from build123d import *
from build123d.topology import SkipClean

# Parameters (mm, degrees)
SKETCH1_R           = 17.5
BOSS_EXTRUDE1_DEPTH = 39
FILLET1_R           = 4.5
SKETCH2_R           = 5
BOSS_EXTRUDE2_DEPTH = 90
SKETCH6_W           = 6
SKETCH6_H           = 26
SKETCH6_W_2         = 14
SKETCH6_W_3         = 18.119457468
SKETCH6_H_2         = 239
SKETCH6_W_4         = 26
SKETCH6_H_3         = 15
SKETCH7_W           = 44.5
SKETCH7_H           = 15
SKETCH8_R           = 28.3
BOSS_EXTRUDE5_DEPTH = 6.5
SKETCH9_R           = 80
BOSS_EXTRUDE6_DEPTH = 1.8
BOSS_EXTRUDE7_START = 13.3
SKETCH10_R          = 8.5
SKETCH10_R_2        = 7.120417841
SKETCH10_R_3        = 5
BOSS_EXTRUDE7_DEPTH = 8
BOSS_EXTRUDE8_START = 21.3
SKETCH10_3_R        = 8.5
SKETCH10_3_R_2      = 7.120417841
SKETCH10_3_R_3      = 5
BOSS_EXTRUDE8_DEPTH = 8
SKETCH14_R          = 28.5
SKETCH14_R_2        = 19.5
BOSS_EXTRUDE9_DEPTH = 26.880542532


with BuildPart() as part:
    # Sketch1 → Boss-Extrude1 (new, symmetric)
    with BuildSketch(Plane(origin=(0, 0, 0), x_dir=(0, 0, -1), z_dir=(1, 0, 0))):
        Circle(SKETCH1_R)
    extrude(amount=BOSS_EXTRUDE1_DEPTH, both=True)

    # Fillet1
    fillet1_edges = [part.edges().sort_by_distance(p)[0] for p in [
        (-39, 0, 17.5),
        (39, 0, 17.5),
    ]]
    fillet(fillet1_edges, radius=FILLET1_R)

    # Sketch2 → Boss-Extrude2 (add, symmetric)
    with BuildSketch(Plane(origin=(0, 0, 0), x_dir=(0, 0, -1), z_dir=(1, 0, 0))):
        with Locations(Location((0, 0, 0), (0, 0, 180))):
            Circle(SKETCH2_R)
    extrude(amount=BOSS_EXTRUDE2_DEPTH, both=True)

    # Sketch6 → Revolve1 (revolve)
    with SkipClean():  # the faces are left unmerged after this step: merging them gives an invalid solid
        with BuildSketch(Plane.XY, mode=Mode.PRIVATE) as revolve1_sk:
            with Locations((-10, 13)):
                Rectangle(SKETCH6_W, SKETCH6_H)
            with Locations((0, 13)):
                Rectangle(SKETCH6_W_2, SKETCH6_H)
            with Locations((10, 13)):
                Rectangle(SKETCH6_W, SKETCH6_H)
            with Locations((-22.059728734, 13)):
                Rectangle(SKETCH6_W_3, SKETCH6_H)
            with Locations((22.059728734, 13)):
                Rectangle(SKETCH6_W_3, SKETCH6_H)
            Polygon((13, 205.545926379), (13, 26), (31.119457468, 26), align=None)
            Polygon((7, 265), (7, 26), (13, 26), (13, 205.545926379), align=None)
            with Locations((0, 145.5)):
                Rectangle(SKETCH6_W_2, SKETCH6_H_2)
            Polygon((-13, 205.545926379), (-13, 26), (-7, 26), (-7, 265), align=None)
            Polygon((-13, 205.545926379), (-31.119457468, 26), (-13, 26), align=None)
            Polygon((-7, 265), (7, 265), (13, 271.5), (-13, 271.5), align=None)
            with Locations((0, 279)):
                Rectangle(SKETCH6_W_4, SKETCH6_H_3)
        revolve(revolve1_sk.sketch.rotate(Axis((-31.119457468, 0, 0), (1, 0, 0)), 90), axis=Axis((-31.119457468, 0, 0), (1, 0, 0)))

    # Sketch7 → Revolve2 (revolve)
    with SkipClean():  # the faces are left unmerged after this step: merging them gives an invalid solid
        with BuildSketch(Plane.XY, mode=Mode.PRIVATE) as revolve2_sk:
            Polygon((22.25, 293.5), (13, 286.5), (-13, 286.5), (-22.25, 293.5), align=None)
            with Locations((0, 301)):
                Rectangle(SKETCH7_W, SKETCH7_H)
            with BuildLine():
                ThreePointArc((-22.25, 308.5), (0, 326.5), (22.25, 308.5))
                Line((22.25, 308.5), (-22.25, 308.5))
            make_face()
        revolve(revolve2_sk.sketch.rotate(Axis((-31.119457468, 0, 0), (1, 0, 0)), 90), axis=Axis((-31.119457468, 0, 0), (1, 0, 0)))

    # Sketch8 → Boss-Extrude5 (add)
    with SkipClean():  # the faces are left unmerged after this step: merging them gives an invalid solid
        with BuildSketch(Plane(origin=(50.5, 0, 0), x_dir=(0, 0, -1), z_dir=(1, 0, 0))):
            Circle(SKETCH8_R)
        extrude(amount=-BOSS_EXTRUDE5_DEPTH)

    # Sketch9 → Boss-Extrude6 (add)
    with SkipClean():  # the faces are left unmerged after this step: merging them gives an invalid solid
        with BuildSketch(Plane(origin=(50.5, 0, 0), x_dir=(0, 0, -1), z_dir=(1, 0, 0))):
            Circle(SKETCH9_R)
        extrude(amount=BOSS_EXTRUDE6_DEPTH)

    # Sketch10 → Boss-Extrude7 (add)
    with SkipClean():  # the faces are left unmerged after this step: merging them gives an invalid solid
        with BuildSketch(Plane(origin=(39, 0, 0), x_dir=(0, 0, -1), z_dir=(1, 0, 0)).offset(BOSS_EXTRUDE7_START)):
            Circle(SKETCH10_R)
            Circle(SKETCH10_R_2, mode=Mode.SUBTRACT)
            Circle(SKETCH10_R_2)
            with Locations(Location((0, 0, 0), (0, 0, 180))):
                Circle(SKETCH10_R_3, mode=Mode.SUBTRACT)
        boss_extrude7 = extrude(amount=BOSS_EXTRUDE7_DEPTH)

    # Sketch10_3 → Boss-Extrude8 (add)
    with SkipClean():  # the faces are left unmerged after this step: merging them gives an invalid solid
        with BuildSketch(Plane(origin=(39, 0, 0), x_dir=(0, 0, -1), z_dir=(1, 0, 0)).offset(BOSS_EXTRUDE8_START)):
            with BuildLine():
                ThreePointArc((-7.361215909, 4.25000004), (-4.24999998, 7.361215944), (0, 8.5))
                Line((0, 8.5), (-4.907477288, 8.5))
                Line((-4.907477288, 8.5), (-7.361215909, 4.25000004))
            make_face()
            with BuildLine():
                ThreePointArc((0, 8.5), (4.250000062, 7.361215896), (7.361216004, 4.249999875))
                Line((7.361216004, 4.249999875), (4.907477288, 8.5))
                Line((4.907477288, 8.5), (0, 8.5))
            make_face()
            with BuildLine():
                ThreePointArc((-7.361215915, -4.250000029), (-8.5, 6e-09), (-7.361215909, 4.25000004))
                Line((-7.361215909, 4.25000004), (-9.814954576, 0))
                Line((-9.814954576, 0), (-7.361215915, -4.250000029))
            make_face()
            with BuildLine():
                Line((-4.907477288, -8.5), (0, -8.5))
                ThreePointArc((0, -8.5), (-4.249999985, -7.361215941), (-7.361215915, -4.250000029))
                Line((-7.361215915, -4.250000029), (-4.907477288, -8.5))
            make_face()
            with BuildLine():
                Line((4.907477288, -8.5), (7.36121598, -4.249999918))
                ThreePointArc((7.36121598, -4.249999918), (4.250000041, -7.361215908), (0, -8.5))
                Line((0, -8.5), (4.907477288, -8.5))
            make_face()
            with BuildLine():
                Line((7.36121598, -4.249999918), (9.814954576, 0))
                Line((9.814954576, 0), (7.361216004, 4.249999875))
                ThreePointArc((7.361216004, 4.249999875), (8.210369542, 2.199961814), (8.5, 0))
                ThreePointArc((8.5, 0), (8.210369536, -2.199961837), (7.36121598, -4.249999918))
            make_face()
            with Locations(Location((0, 0, 0), (0, 0, 210))):
                Circle(SKETCH10_3_R)
            Circle(SKETCH10_3_R_2, mode=Mode.SUBTRACT)
            Circle(SKETCH10_3_R_2)
            with Locations(Location((0, 0, 0), (0, 0, 180))):
                Circle(SKETCH10_3_R_3, mode=Mode.SUBTRACT)
        boss_extrude8 = extrude(amount=BOSS_EXTRUDE8_DEPTH)

    # Mirror2: Boss-Extrude7, Boss-Extrude8 across plane
    with SkipClean():  # the faces are left unmerged after this step: merging them gives an invalid solid
        add(boss_extrude7.mirror(Plane(origin=(0, 0, 0), x_dir=(0, 0, 1), z_dir=(1, 0, 0))))
        add(boss_extrude8.mirror(Plane(origin=(0, 0, 0), x_dir=(0, 0, 1), z_dir=(1, 0, 0))))

    # Sketch14 → Boss-Extrude9 (add)
    with SkipClean():  # the faces are left unmerged after this step: merging them gives an invalid solid
        with BuildSketch(Plane.ZY.offset(58)):
            Circle(SKETCH14_R)
            Circle(SKETCH14_R_2, mode=Mode.SUBTRACT)
        extrude(amount=-BOSS_EXTRUDE9_DEPTH)


solid = part.part
Here's how the part is built. I have some questions about the finished solid (model axes, mm). A direction names the side the tool comes from. Give positions to 0.01 mm unless a question says otherwise; leave off trailing zeros. Use a Markdown table: item, result. Add a question column.
Item 1: If we mould it in two halves opening along Y, with no side actions, what happens to faces 1 (the face through (7.38, 259.1, -57.53)), 2 (the face through (39, 0, -6)), 3 (the face through (47.296, -25.107, -13.059))? For each: pulls with the +Y half, pulls with the -Y half, needs draft (parallel to the pull), parting line crosses it, or undercut.
Item 2: Will these pins go through, and if not, where does the flat tip stop? pin 1 (10 mm diameter, centred on y = -163.5, z = -164.5, fed in from +X); pin 2 (0.7 mm diameter, centred on y = 2, z = -8.5, fed in from -X); pin 3 (4 mm diameter, centred on y = 253.5, z = -100.5, fed in from -X).
Item 3: For faces 4 (the face through (-44.748, 19.334, -2.539)), 5 (the face through (51.39, -78.1, 17.34)), 6 (the face through (-56.244, 7.167, -4.57)), which set-ups out of +Z, -Z, +X, -X, +Y, -Y let a thin tool reach every point of the face, with its end or its side?
Item 4: I need wall thicknesses on line 1 (Y direction, x = -44.5, z = 0); line 2 (X direction, y = -75, z = 284); line 3 (X direction, y = 133.5, z = 93). Which ranges of each line are inside material? Lowest first, please.
Data:
| question | item | result |
|---|---|---|
| 1 | face 1 | undercut |
| 1 | face 2 | needs draft |
| 1 | face 3 | parting line crosses it |
| 2 | pin 1 | stops at x = 10.84 |
| 2 | pin 2 | stops at x = -68.3 |
| 2 | pin 3 | stops at x = -13 |
| 3 | face 4 | -X |
| 3 | face 5 | +X |
| 3 | face 6 | none |
| 4 | line 1 | y = -28.5 to -19.5, -5 to 5, 19.5 to 28.5 |
| 4 | line 2 | x = -22.25 to 22.25 |
| 4 | line 3 | x = -17.32 to 17.32 |
